Input: dimensioned drawing with shaded views. Units: mm. Origin: part minimum x, y, z. A direction names the side the tool comes from. Coordinates: 2 decimals unless noted, no trailing zeros. Order: outer loops, then holes, each group sorted by start corner. A loop starts at its lowest first (then second) coordinate and runs counter-clockwise, first axis right, second up. Notation, with made-up numbers: M -21.5,-0.5 L -9.5,-0.5 A9 ccw -9.5,8.5 Z; hole C 14,-15.5 d6. An arc over 180 degrees is marked long. Use CSV: the item, a comma, the result in double quotes. Start each with the question number.
1. Section query B-B on z = 2.75. Return the cut outline in (x, y), and give its area (3 significant figures).
2. Material intervals for line 1 (X direction, y = 15.5, z = 4); line 2 (X direction, y = 18.5, z = 1.75); line 3 (Y direction, x = 22.5, z = 5.75), sorted ascending.
3. Section query D-D on y = 2.5. Return the cut outline in (x, z) (1 decimal).
4. First-contact query: P1, Ø3.5, axis at x = 75, z = 4.5, coming from the -Y side; P2, Ø3.5, axis at x = 1, z = 3.5, coming from the -Y side; P3, Ø2, axis at x = 44.5, z = 5, coming from the +Y side. Flat tips, straight axial feed; report the tip coordinate or a pass-through.
5. Pull-direction query (X, two-part tool) for the marked faces 3, 4 and 5; classes: pulls with the +X half, pulls with the -X half, needs draft (parallel to the pull), parting line crosses it, or undercut.
6. Section query C-C on x = 38.5. Return the cut outline in (y, z).
7. Set-up query: the marked faces 1 and 2. Return all of +Z, -Z, +X, -X, +Y, -Y with unobstructed straight access to the full face (end or side cutting, diameter ignored); none if empty.
8. Section query A-A on y = 10. Return the cut outline in (x, z).
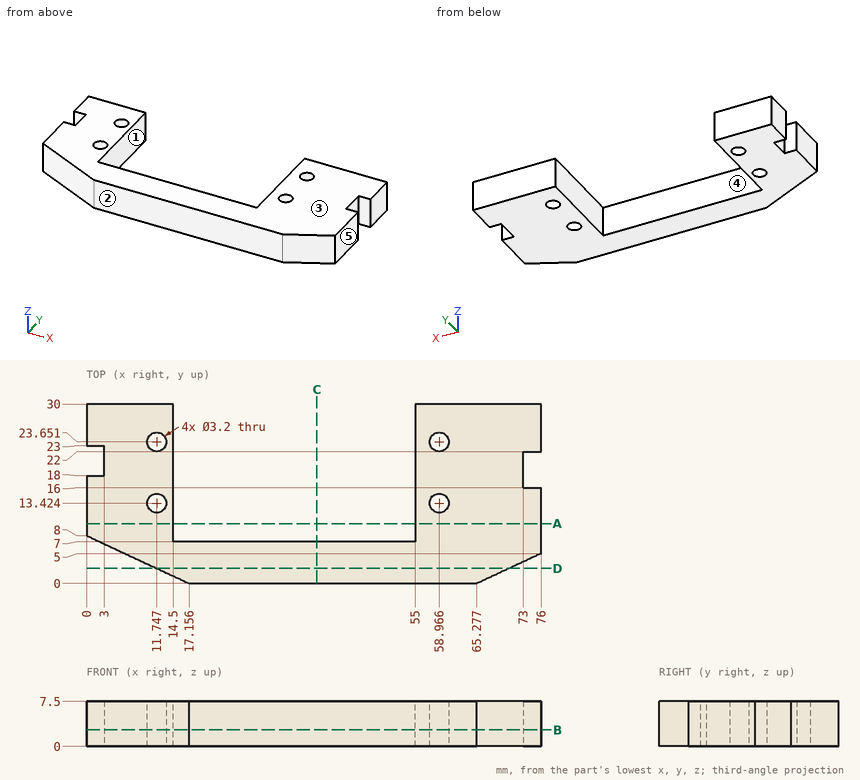
Results list:
1,outline,"M 0,8 L 17.16,0 L 65.28,0 L 76,5 L 76,16 L 73,16 L 73,22 L 76,22 L 76,30 L 55,30 L 55,7 L 14.5,7 L 14.5,30 L 0,30 L 0,23 L 3,23 L 3,18 L 0,18 Z; hole C 11.75,13.42 d3.2; hole C 11.75,23.65 d3.2; hole C 58.97,13.42 d3.2; hole C 58.97,23.65 d3.2"
1,area,"1,190 mm²"
2,line 1,"x = 0 to 14.5, 55 to 76"
2,line 2,"x = 3 to 14.5, 55 to 73"
2,line 3,"y = 0 to 7"
3,outline,"M 11.8,0 L 70.6,0 L 70.6,7.5 L 11.8,7.5 Z"
4,P1,"stops at y = 3.72"
4,P2,"stops at y = 6.72"
4,P3,"stops at y = 7"
5,face 3,"needs draft"
5,face 4,"undercut"
5,face 5,"pulls with the +X half"
6,outline,"M 0,0 L 7,0 L 7,7.5 L 0,7.5 Z"
7,face 1,"+Z, -Z, +Y"
7,face 2,"+Z, -Z, +X, -X, -Y"
8,outline,"M 0,0 L 14.5,0 L 14.5,7.5 L 0,7.5 Z; M 55,0 L 76,0 L 76,7.5 L 55,7.5 Z"
